Verification items for the finished model (mm, model axes). A direction names the side the tool comes from. Round coordinates to 2 decimals unless told otherwise and drop trailing zeros. Write each loop counter-clockwise with the first axis right and the second up, starting at its lowest first coordinate (ties: lowest second). Pieces come first, ordered by that corner, then holes. Notation, with made-up numbers: M 83.5,-5.75 L 129.5,-5.75 A33 ccw 129.5,25.25 Z; hole C 85.5,24.25 d6. An arc over 180 degrees is marked long. Use a Markdown table: item, result. Add a question column.
from build123d import *

# Parameters (mm, degrees)
SKETCH_1_R      = 1.5
EXTRUDE_1_DEPTH = 4
FILLET_2_R      = 0.2


with BuildPart() as part:
    # 草图1 → 凸台-拉伸1 (new body)
    with BuildSketch(Plane(origin=(0, 0, 0), x_dir=(1, 0, 0), z_dir=(0, 1, 0))):
        Polygon((2.305209376, -2.183882567), (3.04390247, 0.904428597), (0.738693094, 3.088311164), (-2.305209376, 2.183882567), (-3.04390247, -0.904428597), (-0.738693094, -3.088311164), align=None)
        Circle(SKETCH_1_R, mode=Mode.SUBTRACT)
    extrude(amount=EXTRUDE_1_DEPTH)

    # 草图2 → 切除-旋转1 (revolve, cut)
    with BuildSketch(Plane.XY):
        Polygon((-4, 2.5), (-2, 3), (-2, 4), (-4, 4), align=None)
    revolve(axis=Axis((0, 4, 0), (0, -1, 0)), mode=Mode.SUBTRACT)

    # 圆角2
    fillet_2_edges = [part.edges().sort_by_distance(p)[0] for p in [
        (-1.5, 4, 0),
        (2, 4, 0),
    ]]
    fillet(fillet_2_edges, radius=FILLET_2_R)


solid = part.part
1. Cross-section at D-D on y = 3.3. Enter the section's corners in (x, z).
2. Cross-section at C-C on x = 0. Enter the section's corners in (y, z), plus the area to 3 significant figures.
3. Cross-section at B-B on z = 0. Enter the section's corners in (x, y), plus the area to 3 significant figures.
4. Depth check by flat-ended pin: pin 1 Ø2 at (x, z) = (-1.5, 0.5) entering from -Y; pin 2 Ø1.8 at (x, z) = (0, 0) entering from +Y. Enter the tip coordinate at first touch or a pass-through.
5. Cross-section at A-A on y = 1.05. Enter the section's corners in (x, z).
6. Scan lines: line 1 along Z through (x, y) = (0, 3.3); line 2 along X through (y, z) = (0.95, 0); line 3 along Z through (x, y) = (-0.5, 0.5). Record each from-to range of solid material in increasing order. Write a range as from..to.
7. Access from +Z, -Z, +X, -X, +Y, -Y to the whole of each face (thin tool, end or side, straight path). Record for faces 1 (the cylindrical face through (0.434, 3.406, 1.952)), 2 (the flat face through (1.91, 1.39, -1.98)).
8. Release check for a two-part mould opening along X. For faces 3 (the flat face through (2.67, 1.39, 0.66)), 4 (the flat face through (-1.91, 1.39, 1.98)), 5 (the cylindrical face through (-1.5, 1.87, -0.07)) record: +X half, -X half, draft (parallel to the pull), parting line (faces both ways), or undercut.
Answer:
| question | item | result |
|---|---|---|
| 1 | outline | C 0,0 d4; hole C 0,0 d3 |
| 2 | outline | M 0,-2.87 L 2.78,-2.87 L 3,-2 L 3.8,-2 A0.2 ccw 4,-1.8 L 4,-1.7 A0.2 ccw 3.8,-1.5 L 0,-1.5 Z; M 0,1.5 L 3.8,1.5 A0.2 ccw 4,1.7 L 4,1.8 A0.2 ccw 3.8,2 L 3,2 L 2.78,2.87 L 0,2.87 Z |
| 2 | area | 8.99 mm^2 |
| 3 | outline | M -2.83,0 L -1.5,0 L -1.5,3.8 A0.2 ccw -1.7,4 L -1.8,4 A0.2 ccw -2,3.8 L -2,3 L -2.83,2.79 Z; M 1.5,0 L 2.83,0 L 2.83,2.79 L 2,3 L 2,3.8 A0.2 ccw 1.8,4 L 1.7,4 A0.2 ccw 1.5,3.8 Z |
| 3 | area | 8.76 mm^2 |
| 4 | pin 1 | stops at y = 0 |
| 4 | pin 2 | passes through |
| 5 | outline | M -3.04,0.9 L -2.31,-2.18 L 0.74,-3.09 L 3.04,-0.9 L 2.31,2.18 L -0.74,3.09 Z; hole C 0,0 d3 |
| 6 | line 1 | z = -2..-1.5, 1.5..2 |
| 6 | line 2 | x = -2.83..-1.5, 1.5..2.83 |
| 6 | line 3 | z = -2.72..-1.41, 1.41..3.02 |
| 7 | face 1 | +Y |
| 7 | face 2 | -Z, +X, +Y, -Y |
| 8 | face 3 | +X half |
| 8 | face 4 | -X half |
| 8 | face 5 | undercut |
